Check sheet for the drawn part. Datum: minimum x, y, z corner. Units: mm. A direction names the side the tool comes from. Coordinates: 2 decimals unless noted, no trailing zeros. Order: outer loops, then holes, each group sorted by start corner. A loop starts at its lowest first (then second) coordinate and runs counter-clockwise, first axis right, second up.
1. Cross-section at C-C (x = 8). Enter the section's corners in (y, z) (1 decimal), then the cut area to 3 significant figures.
2. Set-up check for the marked faces 1, 2, 3 and 4: record each of +Z, -Z, +X, -X, +Y, -Y from which the full face is reachable in a straight line by a thin tool's end or side.
3. Gauge pin test, flat ends, axial feed: pin 1 Ø7.5 at (x, y) = (69.5, 9.5) entering from +Z; pin 2 Ø12.5 at (y, z) = (19, 15) entering from -X; pin 3 Ø7.5 at (x, y) = (64.5, 14) entering from -Z. Record the tip position at first contact, or that the pin passes through.
4. Cross-section at B-B (z = 14). Enter the section's corners in (x, y).
5. Thickness scan on line 1 (X direction, y = 2.5, z = 23.5); line 2 (Z direction, x = 80, y = 18.5) (1 decimal). Record the ranges inside material, lowest first.
6. Cross-section at A-A (y = 18.25). Enter the section's corners in (x, z) (1 decimal).
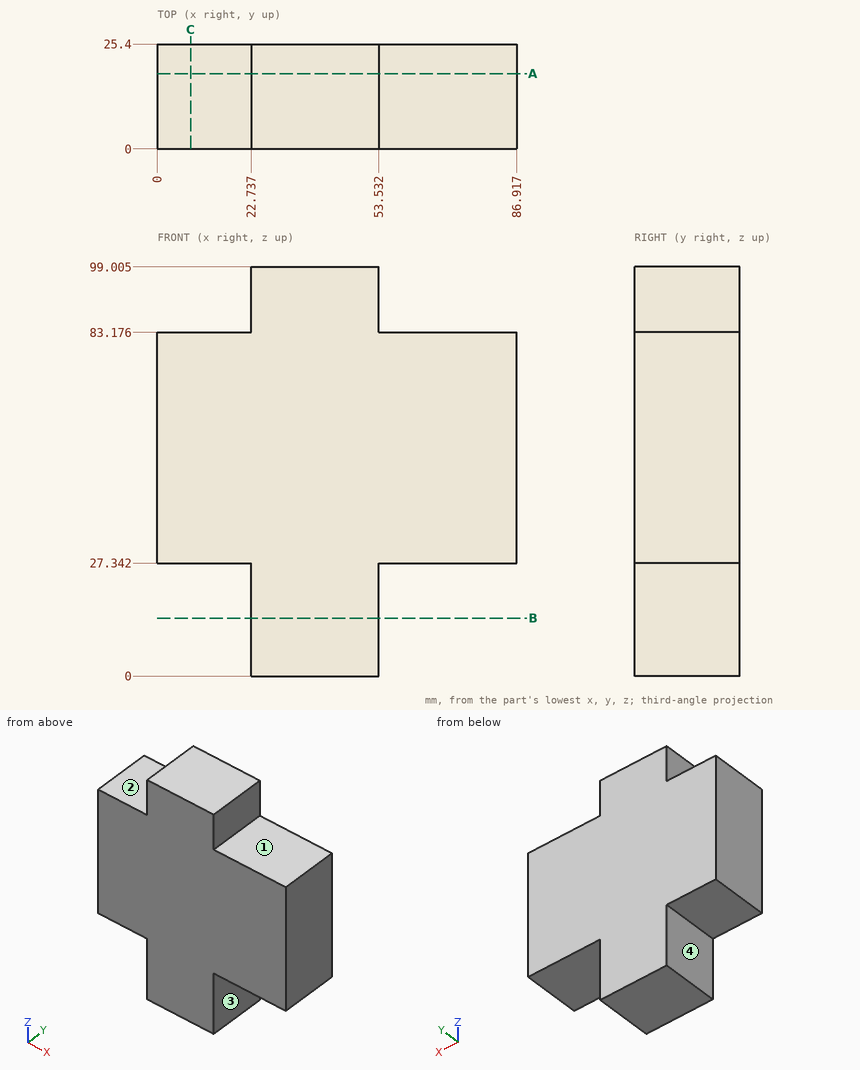
Data:
1. outline: (0, 27.3) - (25.4, 27.3) - (25.4, 83.2) - (0, 83.2) - close
1. area: 1,420 mm2
2. face 1: +Z, +X, +Y, -Y
2. face 2: +Z, -X, +Y, -Y
2. face 3: -Z, +X, +Y, -Y
2. face 4: -Z, -X, +Y, -Y
3. pin 1: stops at z = 83.18
3. pin 2: stops at x = 22.74
3. pin 3: stops at z = 27.34
4. outline: (22.74, 0) - (53.53, 0) - (53.53, 25.4) - (22.74, 25.4) - close
5. line 1: x = 22.74 to 53.53
5. line 2: z = 27.3 to 83.2
6. outline: (0, 27.3) - (22.7, 27.3) - (22.7, 0) - (53.5, 0) - (53.5, 27.3) - (86.9, 27.3) - (86.9, 83.2) - (53.5, 83.2) - (53.5, 99) - (22.7, 99) - (22.7, 83.2) - (0, 83.2) - close
